```python
from build123d import *

# Parameters (mm, degrees)
TABAN_FLAN_1_DEPTH         = 12
KES_EKSTR_ZYON1_DEPTH      = 2662.181692407
KES_EKSTR_ZYON1_DEPTH_BACK = 2662.181692407
IZIM2_W                    = 2500
IZIM2_H                    = 10
KES_EKSTR_ZYON2_DEPTH      = 2662.181692407
KES_EKSTR_ZYON2_DEPTH_BACK = 2662.181692407


# Sheet-metal steps are written as plain solids
with BuildPart() as part:
    # Çizim1 → Taban-Flanş1 (new body)
    with BuildSketch(Plane.XY):
        Polygon((0, 0), (0, 795), (660, 912), (1840, 912), (2500, 795), (2500, 0), align=None)
    extrude(amount=-TABAN_FLAN_1_DEPTH)

    # Çizim2 → Kes-Ekstrüzyon1 (cut, two sides: drawn at the far end of the back side and taken through both)
    with BuildSketch(Plane.XY.offset(-KES_EKSTR_ZYON1_DEPTH_BACK)):
        with Locations((1250, 5)):
            Rectangle(IZIM2_W, IZIM2_H)
    extrude(amount=KES_EKSTR_ZYON1_DEPTH + KES_EKSTR_ZYON1_DEPTH_BACK, mode=Mode.SUBTRACT)

    # Çizim3 → Kes-Ekstrüzyon2 (cut, two sides: drawn at the far end of the back side and taken through both)
    with BuildSketch(Plane.XY.offset(-KES_EKSTR_ZYON2_DEPTH_BACK)):
        Polygon((810, 10), (810, 912), (-172.469977519, 1159.159604292), (-279.270596873, -118.492249454), (448.555846128, -150.136877411), align=None)
    extrude(amount=KES_EKSTR_ZYON2_DEPTH + KES_EKSTR_ZYON2_DEPTH_BACK, mode=Mode.SUBTRACT)


solid = part.part
```
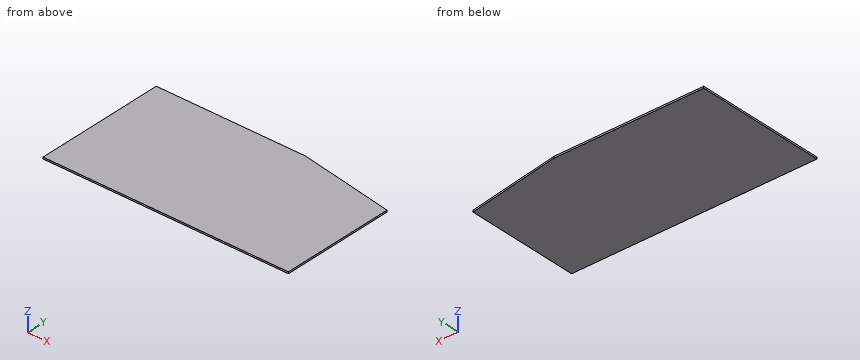
Model file for the job. Use its own axes, mm. Give positions to 0.01 mm unless a question says otherwise; leave off trailing zeros. Write each loop counter-clockwise with the first axis right and the second up, starting at its lowest first coordinate (ties: lowest second). Pieces come first, ordered by that corner, then holes. Notation, with made-up numbers: M -5,-12.75 L 27,-12.75 A19 cw 27,17.25 Z; hole C 23.25,85.5 d8. An arc over 180 degrees is marked long. Use a Markdown table: item, result.
1) Cut at C-C (x = 2299.5). List the corners of the cut face in (y, z), and give its area (3 significant figures).
Responses:
| item | result |
|---|---|
| outline | M 10,-12 L 830.54,-12 L 830.54,0 L 10,0 Z |
| area | 9,850 mm2 |
2) Cut at A-A (z = -9). List the corners of the cut face in (x, y), and give its area (3 significant figures).
Responses:
| item | result |
|---|---|
| outline | M 810,10 L 2500,10 L 2500,795 L 1840,912 L 810,912 Z |
| area | 1,490,000 mm2 |
3) Cut at B-B (y = 814.5). List the corners of the cut face in (x, z).
Responses:
| item | result |
|---|---|
| outline | M 810,-12 L 2390,-12 L 2390,0 L 810,0 Z |
4) Drill centre line: line 1 (Y direction, x = 2060, z = -9.25). Where is it in solid material? Low to high. Write a range as from..to.
Responses:
| item | result |
|---|---|
| line 1 | y = 10..873 |
5) Pin check, flat tips, straight feed: pin 1 (5 mm diameter, centred on x = 1037.5, y = 737, fed in from +Z); pin 2 (3 mm diameter, centred on x = 2038, z = -9, fed in from +Y). Stop position of each tip, or through.
Responses:
| item | result |
|---|---|
| pin 1 | stops at z = 0 |
| pin 2 | stops at y = 877.17 |
